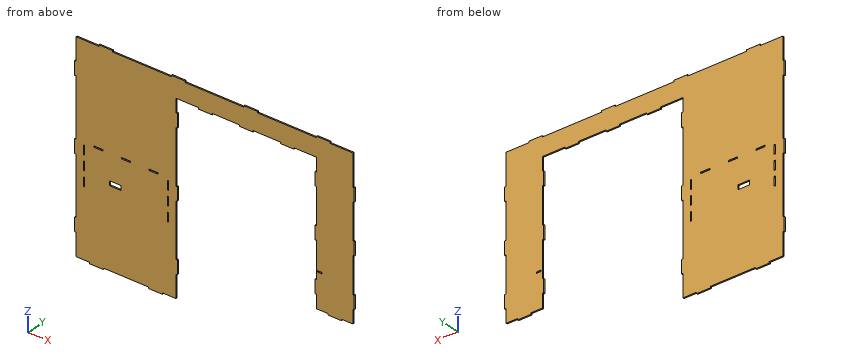
```python
from build123d import *

# Parameters (mm, degrees)
SKETCH1_W           = 3
SKETCH1_H           = 20
SKETCH1_W_2         = 20
SKETCH1_H_2         = 3
BOSS_EXTRUDE1_DEPTH = 3
SKETCH2_W           = 10
SKETCH2_H           = 3
SKETCH2_W_2         = 25
SKETCH2_H_2         = 10
CUT_EXTRUDE1_DEPTH  = 10


with BuildPart() as part:
    # Sketch1 → Boss-Extrude1 (new body)
    with BuildSketch(Plane(origin=(0, 0, 0), x_dir=(1, 0, 0), z_dir=(0, 1, 0))):
        Polygon((0, 0), (0, 50), (-3, 50), (-3, 80), (0, 80), (0, 210), (-3, 210), (-3, 240), (0, 240), (0, 370), (-3, 370), (-3, 400), (0, 400), (0, 450), (30, 450), (30, 453), (60, 453), (60, 450), (160, 450), (160, 453), (190, 453), (190, 450), (220, 450), (220, 400), (223, 400), (223, 370), (220, 370), (220, 250), (223, 250), (223, 220), (220, 220), (220, 100), (223, 100), (223, 70), (220, 70), (220, 40), (270, 40), (270, 43), (300, 43), (300, 40), (360, 40), (360, 43), (390, 43), (390, 40), (450, 40), (450, 43), (480, 43), (480, 40), (530, 40), (530, 70), (527, 70), (527, 100), (530, 100), (530, 180), (527, 180), (527, 210), (530, 210), (530, 290), (527, 290), (527, 320), (530, 320), (530, 350), (555, 350), (555, 353), (585, 353), (585, 350), (610, 350), (610, 320), (613, 320), (613, 290), (610, 290), (610, 210), (613, 210), (613, 180), (610, 180), (610, 100), (613, 100), (613, 70), (610, 70), (610, 0), (560, 0), (560, -3), (530, -3), (530, 0), (400, 0), (400, -3), (370, -3), (370, 0), (240, 0), (240, -3), (210, -3), (210, 0), (80, 0), (80, -3), (50, -3), (50, 0), align=None)
        with Locations((17.5, 225)):
            Rectangle(SKETCH1_W, SKETCH1_H, mode=Mode.SUBTRACT)
        with Locations((17.5, 257.5)):
            Rectangle(SKETCH1_W, SKETCH1_H, mode=Mode.SUBTRACT)
        with Locations((17.5, 290)):
            Rectangle(SKETCH1_W, SKETCH1_H, mode=Mode.SUBTRACT)
        with Locations((49, 209.5)):
            Rectangle(SKETCH1_W_2, SKETCH1_H_2, mode=Mode.SUBTRACT)
        with Locations((110, 209.5)):
            Rectangle(SKETCH1_W_2, SKETCH1_H_2, mode=Mode.SUBTRACT)
        with Locations((171, 209.5)):
            Rectangle(SKETCH1_W_2, SKETCH1_H_2, mode=Mode.SUBTRACT)
        with Locations((202.5, 225)):
            Rectangle(SKETCH1_W, SKETCH1_H, mode=Mode.SUBTRACT)
        with Locations((202.5, 257.5)):
            Rectangle(SKETCH1_W, SKETCH1_H, mode=Mode.SUBTRACT)
        with Locations((202.5, 290)):
            Rectangle(SKETCH1_W, SKETCH1_H, mode=Mode.SUBTRACT)
    extrude(amount=BOSS_EXTRUDE1_DEPTH)

    # Sketch2 → Cut-Extrude1 (cut)
    with BuildSketch(Plane(origin=(0, 3, 0), x_dir=(1, 0, 0), z_dir=(0, 1, 0))):
        with Locations((537.5, 272.5)):
            Rectangle(SKETCH2_W, SKETCH2_H)
        with Locations((86.5, 271)):
            Rectangle(SKETCH2_W_2, SKETCH2_H_2)
    extrude(amount=-CUT_EXTRUDE1_DEPTH, mode=Mode.SUBTRACT)


solid = part.part
```
The model under review builds one solid part; all positions refer to its coordinate system, in mm. Coordinates: 2 decimals unless noted, no trailing zeros. Order: outer loops, then holes, each group sorted by start corner. A loop starts at its lowest first (then second) coordinate and runs counter-clockwise, first axis right, second up. Notation, with made-up numbers: (-3, 31.25) -> (4, 31.25) arc R9 ccw to (4, 42.25) -> close; hole circle Ø7 at (-35.75, -30.75). An arc over 180 degrees is marked (long way). Answer in a Markdown table with one row per item. Add a question column.
Item 1: We need section B-B on y = 1.6. Give the number of separate pieces and of enclosed holes in the cut face, plus the area to 3 significant figures.
Item 2: We need section A-A on z = -193.5. Write out the cut boundary in (x, y).
Item 3: We need section D-D on z = -390. Write out the cut boundary in (x, y), plus the area to 3 significant figures.
Item 4: Clearance check with flat-ended pins moving along their axes: pin 1 (1.5 mm diameter, centred on x = 151.5, y = 0.5, fed in from +Z); pin 2 (1.5 mm diameter, centred on x = 466.5, y = 1, fed in from -Z); pin 3 (0.9 mm diameter, centred on y = 2, z = -271, fed in from -X). State where each tip first meets the part, or that it passes through.
Item 5: We need section C-C on x = 346. Write out the cut boundary in (y, z).
Item 6: To check wall thickness, follow probe 1 along Z at (x, y) = (39.5, 1.65); probe 2 along X at (y, z) = (0.7, -116); probe 3 along X at (y, z) = (0.55, -87.5). State the ranges of each line that lie inside material, in increasing order.
Final values:
| question | item | result |
|---|---|---|
| 1 | separate pieces | 1 |
| 1 | enclosed holes | 11 |
| 1 | area | 141,000 mm2 |
| 2 | outline | (0, 0) -> (220, 0) -> (220, 3) -> (0, 3) -> close; (527, 0) -> (613, 0) -> (613, 3) -> (527, 3) -> close |
| 3 | outline | (-3, 0) -> (223, 0) -> (223, 3) -> (-3, 3) -> close |
| 3 | area | 678 mm2 |
| 4 | pin 1 | stops at z = 0 |
| 4 | pin 2 | stops at z = -43 |
| 4 | pin 3 | stops at x = 0 |
| 5 | outline | (0, -40) -> (3, -40) -> (3, 0) -> (0, 0) -> close |
| 6 | probe 1 | z = -453 to -211, -208 to 0 |
| 6 | probe 2 | x = 0 to 220, 530 to 610 |
| 6 | probe 3 | x = 0 to 223, 527 to 613 |
